Drawing for the job (mm, zero at the part's lowest x, y, z). A direction names the side the tool comes from. Coordinates: 2 decimals unless noted, no trailing zeros. Order: outer loops, then holes, each group sorted by start corner. A loop starts at its lowest first (then second) coordinate and runs counter-clockwise, first axis right, second up.
1) Cut at B-B (x = 40). List the corners of the cut face in (y, z), and give its area (3 significant figures).
2) Cut at C-C (y = 48). List the corners of the cut face in (x, z).
3) Pin check, flat tips, straight feed: pin 1 Ø12 at (x, y) = (28.5, 38.5) entering from -Z; pin 2 Ø2 at (x, z) = (15, 68) entering from +Y. Stop position of each tip, or through.
4) Cut at D-D (z = 10.5). List the corners of the cut face in (x, y).
5) Wall check: L1, parallel to Y at x = 23, z = 24; L2, parallel to Z at x = 51, y = 55; L3, parallel to X at y = 44, z = 46.5. Give the ranges that are in metal, low to high.
6) Tool access for the marked faces 1 and 2: list every direction of +Z, -Z, +X, -X, +Y, -Y with a clear straight run to the whole face (end or side of a thin tool).
7) Cut at A-A (z = 40). List the corners of the cut face in (x, y).
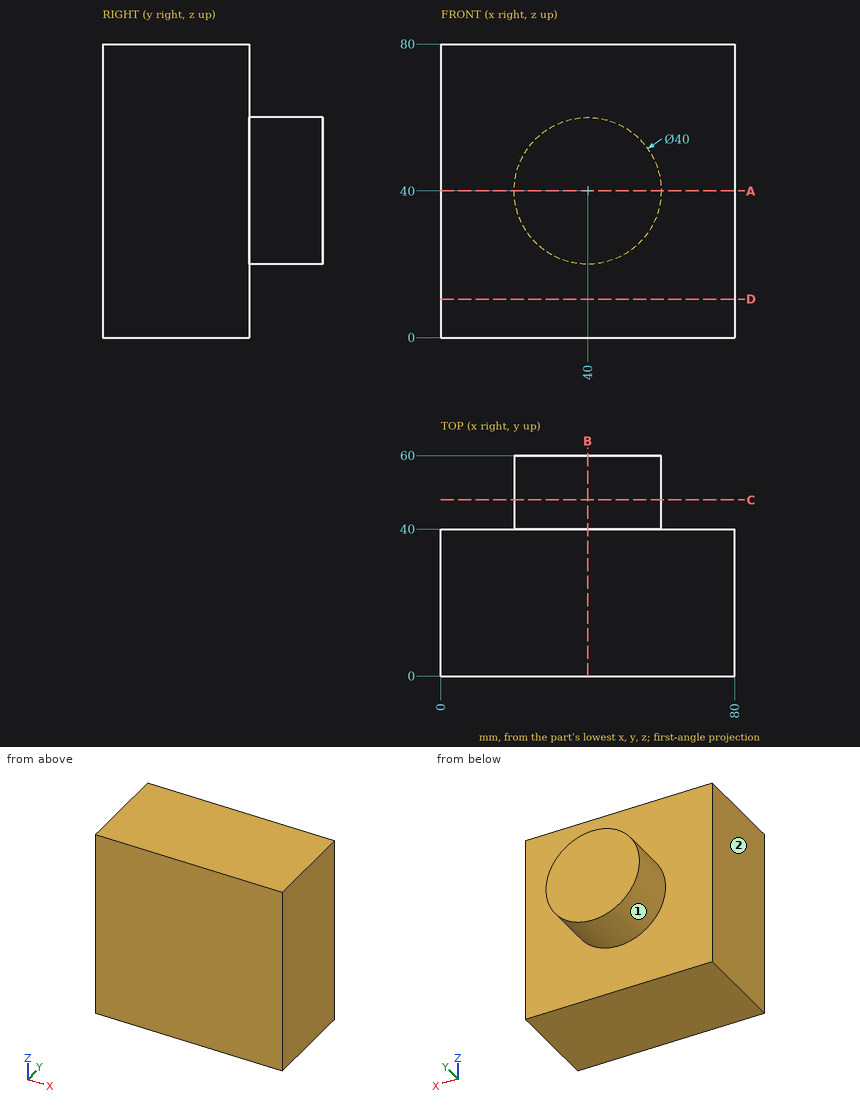
Geometry check:
1. outline: (0, 0) - (40, 0) - (40, 20) - (60, 20) - (60, 60) - (40, 60) - (40, 80) - (0, 80) - close
1. area: 4,000 mm2
2. outline: circle Ø40 at (40, 40)
3. pin 1: stops at z = 0
3. pin 2: stops at y = 40
4. outline: (0, 0) - (80, 0) - (80, 40) - (0, 40) - close
5. L1: y = 0 to 40
5. L2: z = 23.3 to 56.7
5. L3: x = 21.09 to 58.91
6. face 1: +Y
6. face 2: +Z, -Z, -X, +Y, -Y
7. outline: (0, 0) - (80, 0) - (80, 40) - (60, 40) - (60, 60) - (20, 60) - (20, 40) - (0, 40) - close
